Autodesk Inventor part; units mm, degrees
ref_plane "YZ Plane" through (0, 0, 0) normal (1, 0, 0) x (0, 1, 0)
ref_plane "XZ Plane" through (0, 0, 0) normal (0, 1, 0) x (-1, 0, 0)
ref_plane "XY Plane" through (0, 0, 0) normal (0, 0, 1) x (1, 0, 0)
sketch "Sketch1" plane through (0, 0, 0) normal (0, 0, 1) x (1, 0, 0)
  line L0 (-5.3279, 7.3898) -> (14.6721, 7.3898)
  line L1 (14.6721, 7.3898) -> (14.6721, -12.6102)
  line L2 (14.6721, -12.6102) -> (-5.3279, -12.6102)
  line L3 (-5.3279, -12.6102) -> (-5.3279, 7.3898)
  line L4 (-6.3279, 8.3898) -> (15.6721, 8.3898)
  line L5 (15.6721, 8.3898) -> (15.6721, -13.6102)
  line L6 (15.6721, -13.6102) -> (-6.3279, -13.6102)
  line L7 (-6.3279, -13.6102) -> (-6.3279, 8.3898)
  point P0 (0, 0)
  dimension "d0" = 20
  dimension "d1" = 20
  dimension "d2" = 22
  dimension "d3" = 22
  dimension "d4" = 1
  dimension "d5" = 1
extrude "Extrusion1" add sketch "Sketch1" along normal blind 3
sketch "Sketch2" plane through (0, 0, 3) normal (0, 0, 1) x (1, 0, 0)
  line L0 (15.6721, 8.3898) -> (-6.3279, 8.3898)
  line L1 (-6.3279, -13.6102) -> (15.6721, -13.6102)
  line L2 (15.6721, -13.6102) -> (15.6721, 8.3898)
  line L3 (15.6721, 8.3898) -> (-6.3279, 8.3898)
  line L4 (-6.3279, 8.3898) -> (-6.3279, -13.6102)
  point P0 (0, 0)
extrude "Extrusion2" add sketch "Sketch2" along normal blind 1
properties part number "sensor_cover"
The listing builds one solid part. Answer for the finished solid, in the listing's coordinates (mm). A direction names the side the tool comes from. Coordinates: 2 decimals unless noted, no trailing zeros. Write each loop counter-clockwise with the first axis right and the second up, starting at its lowest first coordinate (ties: lowest second). Pieces come first, ordered by that corner, then holes. Notation, with made-up numbers: M 65.25,-18 L 97.25,-18 A23 ccw 97.25,0 Z; hole C 43.25,-17 d8. An arc over 180 degrees is marked long. Use one line per item in the form item = value.
Item 1: Given P1, Ø10, axis at x = 0.5, y = -0.5, coming from the -Z side, flat-ended and moving along its own axis, determine where the tip first touches the part or whether it passes through.
Model answer:
P1 = 3
Item 2: Find section C-C, the plane x = 11.75. Give the vertices of the cut face in (y, z), plus the area to 3 significant figures.
Model answer:
outline = M -13.61,0 L -12.61,0 L -12.61,3 L 7.39,3 L 7.39,0 L 8.39,0 L 8.39,4 L -13.61,4 Z
area = 28.0 mm2
Item 3: For faces 4 (the face through (-5.328, -3, 1)), 5 (the face through (5, -2, 4)), determine the directions among +Z, -Z, +X, -X, +Y, -Y from which every point of the face is accessible in a straight line to the end or side of a thin tool.
Model answer:
face_4 = -Z
face_5 = +Z, +X, -X, +Y, -Y
Item 4: Find section B-B, the plane y = -9. Give the vertices of the cut face in (x, z), plus the area to 3 significant figures.
Model answer:
outline = M -6.33,0 L -5.33,0 L -5.33,3 L 14.67,3 L 14.67,0 L 15.67,0 L 15.67,4 L -6.33,4 Z
area = 28.0 mm2
Item 5: Find section A-A, the plane z = 1. Give the vertices of the cut face in (x, y).
Model answer:
outline = M -6.33,-13.61 L 15.67,-13.61 L 15.67,8.39 L -6.33,8.39 Z; hole M -5.33,-12.61 L 14.67,-12.61 L 14.67,7.39 L -5.33,7.39 Z
Item 6: Find the intervals of material crossed by probe 1 along X at (y, z) = (-11.75, 0.35); probe 2 along Y at (x, z) = (-2.25, 0.35); probe 3 along Z at (x, y) = (-2.75, -0.25), in increasing order.
Model answer:
probe_1 = -6.33 to -5.33, 14.67 to 15.67
probe_2 = -13.61 to -12.61, 7.39 to 8.39
probe_3 = 3 to 4
Item 7: The mould has two halves that part along Y. Classify faces 1 (the face through (5, 8.39, 2)), 2 (the face through (4, -13, 0)), 3 (the face through (5, -12.61, 1)): released by +Y, released by -Y, zero draft, split by the parting line, or undercut.
Model answer:
face_1 = released by +Y
face_2 = zero draft
face_3 = undercut
